from build123d import *

# Parameters (mm, degrees)
BOSS_EXTRUDE1_DEPTH = 28
BOSS_EXTRUDE2_DEPTH = 18
SKETCH2_R           = 3
BOSS_EXTRUDE3_DEPTH = 6


with BuildPart() as part:
    # Sketch1 → Boss-Extrude1 (new body)
    with BuildSketch(Plane.XY):
        Polygon((0, 0), (78, 0), (76.568001833, 46.166688671), (69.317539536, 49.547634765), (54.103282114, 16.920554432), (49.571743179, 19.033645741), (64.786000601, 51.660726074), (51.191383796, 58), (27.876000888, 8), (0, 8), align=None)
    extrude(amount=BOSS_EXTRUDE1_DEPTH)

    # Sketch1<3> → Boss-Extrude2 (add)
    with BuildSketch(Plane.XY):
        Polygon((0, 16), (0, 8), (27.876000888, 8), (40, 34), (24, 34), (24, 16), align=None)
    extrude(amount=BOSS_EXTRUDE2_DEPTH)

    # Sketch2 → Boss-Extrude3 (add)
    with BuildSketch(Plane(origin=(31.358387135, 67.248278227, 0), x_dir=(0.9063077870366482, -0.4226182617407034, 0), z_dir=(0.4226182617407034, 0.9063077870366482, 0))):
        with Locations((29.383290582, -7)):
            Circle(SKETCH2_R)
        with Locations((29.383290582, -21)):
            Circle(SKETCH2_R)
    extrude(amount=BOSS_EXTRUDE3_DEPTH)


solid = part.part
Can you work these out from the model? Positions are in its coordinate system, mm. A direction names the side the tool comes from. Round coordinates to 2 decimals unless told otherwise and drop trailing zeros. Write each loop counter-clockwise with the first axis right and the second up, starting at its lowest first coordinate (ties: lowest second). Pieces come first, ordered by that corner, then holes. Notation, with made-up numbers: (34, 21) - (72, 21) arc R17 ccw to (72, 37) - close; hole circle Ø2 at (36.25, 50.5). An arc over 180 degrees is marked (long way). Write each question's results on one line, items separated by ' | '. Start each with the question number.
1) Which directions (+Z, -Z, +X, -X, +Y, -Y) give clear straight access to the entire face, cutting with the end or side of a thin tool? Please do faces 4 (the flat face through (57.072, 35.119, 13.804)), 5 (the flat face through (24.2, 18.3, 18)), 6 (the flat face through (32, 34, 9)).
2) Suppose I cut it at B-B (y = 48). List the corners of the cut face in (x, z) for me.
3) For pin 1 Ø6 at (x, z) = (14, 6.5) entering from +Y; pin 2 Ø3 at (x, z) = (18.5, 23.5) entering from +Y; pin 3 Ø8 at (y, z) = (14, 13.5) entering from +X; pin 4 Ø13 at (x, y) = (14, 24.5) entering from +Z, each with a flat end and sliding along its axis, tell me the tip position at first contact or that it passes through.
4) Please list where these lines run through material, in increasing order: line 1 (Z direction, x = 58.5, y = 55.5); line 2 (Z direction, x = 36, y = 30); line 3 (Y direction, x = 24.5, z = 24.5).
5) Suppose I cut it at D-D (y = 30). List the corners of the cut face in (x, z) for me.
6) Suppose I cut it at A-A (z = 15.5). List the corners of the cut face in (x, y) for me.
7) Suppose I cut it at C-C (x = 16). List the corners of the cut face in (y, z) for me, and give its area (3 significant figures).
8) We'd pull the mould along X, two halves only. Please class faces 1 (the flat face through (24, 25, 9)), 2 (the cylindrical face through (56.523, 58.778, 6.868)), 3 (the flat face through (60.486, 60.286, 20.958)): released by +X, released by -X, zero draft, split by the parting line, or undercut.
Here are the results:
1) face 4: +Z, -Z | face 5: +Z, -X, +Y | face 6: +Z, -Z, -X, +Y
2) outline: (46.53, 0) - (63.08, 0) - (63.08, 28) - (46.53, 28) - close; (68.6, 0) - (72.64, 0) - (72.64, 28) - (68.6, 28) - close
3) pin 1: stops at y = 16 | pin 2: stops at y = 8 | pin 3: stops at x = 77.69 | pin 4: passes through
4) line 1: z = 4.01 to 9.99, 18.01 to 23.99 | line 2: z = 0 to 18 | line 3: y = 0 to 8
5) outline: (24, 0) - (54.69, 0) - (54.69, 28) - (38.13, 28) - (38.13, 18) - (24, 18) - close; (60.2, 0) - (77.07, 0) - (77.07, 28) - (60.2, 28) - close
6) outline: (0, 0) - (78, 0) - (76.57, 46.17) - (69.32, 49.55) - (54.1, 16.92) - (49.57, 19.03) - (64.79, 51.66) - (51.19, 58) - (40, 34) - (24, 34) - (24, 16) - (0, 16) - close
7) outline: (0, 0) - (16, 0) - (16, 18) - (8, 18) - (8, 28) - (0, 28) - close | area: 368 mm2
8) face 1: released by -X | face 2: undercut | face 3: released by +X
